```python
from build123d import *

# Parameters (mm, degrees)
SKETCH2_R           = 1.55
BOSS_EXTRUDE1_DEPTH = 1
FILLET1_R           = 10
FILLET2_R           = 2
FILLET3_R           = 1


with BuildPart() as part:
    # Sketch2 → Boss-Extrude1 (new body)
    # profile 1 of 2: a face of its own
    with BuildSketch(Plane(origin=(0, 0, 0), x_dir=(1, 0, 0), z_dir=(0, 1, 0))):
        with BuildLine():
            Line((-13.75, 26), (-13.75, 3))
            Line((-13.75, 3), (15.25, 3))
            ThreePointArc((15.25, 3), (17.371320344, 2.121320344), (18.25, 0))
            Line((18.25, 0), (18.25, 26))
            Line((18.25, 26), (-13.75, 26))
        make_face()
        Polygon((2.25, 11.8), (10.25, 5), (-5.75, 5), align=None, mode=Mode.SUBTRACT)
        Polygon((-9.75, 7), (-9.75, 22), (-0.926470588, 14.5), align=None, mode=Mode.SUBTRACT)
        Polygon((5.426470588, 14.5), (14.25, 22), (14.25, 7), align=None, mode=Mode.SUBTRACT)
        Polygon((-5.75, 24), (10.25, 24), (2.25, 17.2), align=None, mode=Mode.SUBTRACT)
    # profile 2 of 2: a face of its own
    with BuildSketch(Plane(origin=(0, 0, 0), x_dir=(1, 0, 0), z_dir=(0, 1, 0))):
        with BuildLine():
            ThreePointArc((15.25, -3), (13.128679656, -2.121320344), (12.25, 0))
            Line((12.25, 0), (-12.25, 0))
            ThreePointArc((-12.25, 0), (-13.128679656, -2.121320344), (-15.25, -3))
            ThreePointArc((-15.25, -3), (-18.25, 0), (-15.25, 3))
            Line((-15.25, 3), (15.25, 3))
            ThreePointArc((15.25, 3), (18.25, 0), (15.25, -3))
        make_face()
        with Locations(Location((15.25, 0, 0), (0, 0, 270))):
            Circle(SKETCH2_R, mode=Mode.SUBTRACT)
        with Locations(Location((-15.25, 0, 0), (0, 0, 270))):
            Circle(SKETCH2_R, mode=Mode.SUBTRACT)
    extrude(amount=BOSS_EXTRUDE1_DEPTH)

    # Fillet1
    fillet1_edges = [part.edges().sort_by_distance(p)[0] for p in [
        (-13.75, 0.5, -3),
        (12.25, 0.5, 0),
        (-12.25, 0.5, 0),
    ]]
    fillet(fillet1_edges, radius=FILLET1_R)

    # Fillet2
    fillet2_edges = [part.edges().sort_by_distance(p)[0] for p in [
        (-13.75, 0.5, -26),
        (18.25, 0.5, -26),
    ]]
    fillet(fillet2_edges, radius=FILLET2_R)

    # Fillet3
    fillet3_edges = [part.edges().sort_by_distance(p)[0] for p in [
        (-5.75, 0.5, -5),
        (10.25, 0.5, -5),
        (2.25, 0.5, -11.8),
        (-9.75, 0.5, -22),
        (-9.75, 0.5, -7),
        (-0.926470588, 0.5, -14.5),
        (14.25, 0.5, -22),
        (5.426470588, 0.5, -14.5),
        (14.25, 0.5, -7),
        (10.25, 0.5, -24),
        (-5.75, 0.5, -24),
        (2.25, 0.5, -17.2),
    ]]
    fillet(fillet3_edges, radius=FILLET3_R)


solid = part.part
```
The listing builds one solid part. Answer for the finished solid, in the listing's coordinates (mm). A direction names the side the tool comes from. Give positions to 0.01 mm unless a question says otherwise; leave off trailing zeros. Order: outer loops, then holes, each group sorted by start corner. A loop starts at its lowest first (then second) coordinate and runs counter-clockwise, first axis right, second up. Notation, with made-up numbers: (-37.75, 14.25) -> (10.25, 14.25) arc R25 ccw to (10.25, 38.25) -> close; hole circle Ø6 at (-3.5, 18.25). An arc over 180 degrees is marked (long way). Answer as a JSON object with one key per item and string values. Group by question number.
Item 1: Consider L1, parallel to Z at x = 2, y = 0.5; L2, parallel to Z at x = -1, y = 0.35; L3, parallel to X at y = 0.3, z = -5.25. Determine where each line is inside the solid, lowest interval first. Write a range as from..to.
Item 2: The part is cut by section C-C on y = 0.7. Give the number of separate pieces and of enclosed holes in the cut face, and give its area (3 significant figures).
Item 3: The part is cut by section A-A on z = -19. Write down the section's boundary in (x, y), and give its area (3 significant figures).
Item 4: The part is cut by section B-B on z = -16. Write down the section's boundary in (x, y).
Item 5: Determine the mould class of faces 3 (the flat face through (0.1, 0.5, 0)), 4 (the flat face through (2.2, 0.5, -24)), 5 (the cylindrical face through (17.68, 0.51, -25.4)), 6 (the flat face through (0, 0, -12)) for opening direction Z: pulls with the +Z half, pulls with the -Z half, needs draft (parallel to the pull), parting line crosses it, or undercut.
Item 6: A tool of negligible diameter and unlimited length cuts with its end or side. For faces 1 (the cylindrical face through (-10.295, 0.507, 0.578)), 2 (the flat face through (9.419, 0.493, -17.893)), from which of +Z, -Z, +X, -X, +Y, -Y can it reach the whole face along a straight path? Write none if from no direction.
Item 7: The part is cut by section D-D on x = -10.5. Write down the section's boundary in (y, z), and give its area (3 significant figures).
Item 8: Flat-ended cylindrical pins translate along their axes: pin 1 (12 mm diameter, centred on x = -5, z = -17, fed in from -Y); pin 2 (1.9 mm diameter, centred on x = 15.25, z = 0, fed in from +Y); pin 3 (0.5 mm diameter, centred on x = -1.5, y = 0.5, fed in from +Z). Find the tip coordinate at first contact, or state that the pin passes through.
Result set:
{
 "1": {"L1": "-26..-24, -17.54..-11.46, -5..0", "L2": "-26..-24, -19.96..-9.04, -5..0", "L3": "-14.86..-3.69, 8.19..18.25"},
 "2": {"separate pieces": "1", "enclosed holes": "6", "area": "637 mm²"},
 "3": {"outline": "(-13.75, 0) -> (-9.75, 0) -> (-9.75, 1) -> (-13.75, 1) -> close; (-6.22, 0) -> (0.13, 0) -> (0.13, 1) -> (-6.22, 1) -> close; (4.37, 0) -> (10.72, 0) -> (10.72, 1) -> (4.37, 1) -> close; (14.25, 0) -> (18.25, 0) -> (18.25, 1) -> (14.25, 1) -> close", "area": "20.7 mm²"},
 "4": {"outline": "(-13.75, 0) -> (-9.75, 0) -> (-9.75, 1) -> (-13.75, 1) -> close; (-2.69, 0) -> (7.19, 0) -> (7.19, 1) -> (-2.69, 1) -> close; (14.25, 0) -> (18.25, 0) -> (18.25, 1) -> (14.25, 1) -> close"},
 "5": {"face 3": "pulls with the +Z half", "face 4": "undercut", "face 5": "pulls with the -Z half", "face 6": "needs draft"},
 "6": {"face 1": "+Z, +Y, -Y", "face 2": "+Y, -Y"},
 "7": {"outline": "(0, -26) -> (1, -26) -> (1, 0.65) -> (0, 0.65) -> close", "area": "26.7 mm²"},
 "8": {"pin 1": "y = 0", "pin 2": "through", "pin 3": "z = 0"}
}
